Geometry: final body of the model. Coordinates: model frame, mm. Face numbers are marked on the shaded views. A direction names the side the tool comes from. Give positions to 0.01 mm unless a question says otherwise; leave off trailing zeros. Order: outer loops, then holes, each group sorted by start corner. A loop starts at its lowest first (then second) coordinate and runs counter-clockwise, first axis right, second up. Notation, with made-up numbers: M 79.25,-20 L 104.25,-20 A24 cw 104.25,12 Z; hole C -33,-0.5 d9. An arc over 180 degrees is marked long. Use CSV: the item, a comma, the result in double quotes.
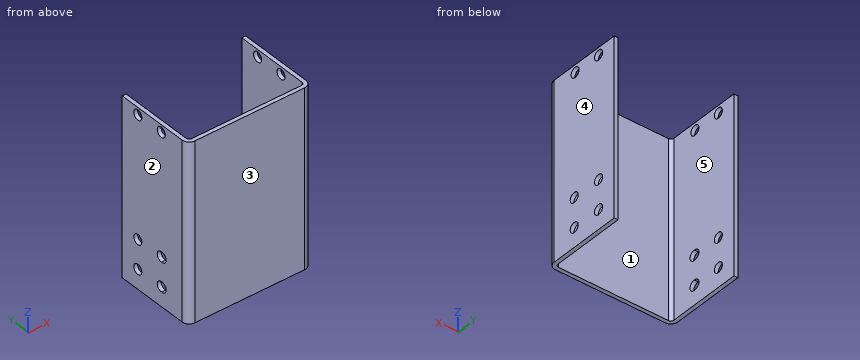
```python
from build123d import *

# Parameters (mm, degrees)
EXTRUDE_THIN1_DEPTH        = 57.935499968
F_4_CLEARANCE_HOLE1_REACH  = 115.405
F_4_CLEARANCE_HOLE1_BORE_R = 1.63195
F_4_CLEARANCE_HOLE2_D      = 3.2639
F_4_CLEARANCE_HOLE3_REACH  = 115.405
F_4_CLEARANCE_HOLE3_BORE_R = 1.63195
F_4_CLEARANCE_HOLE4_D      = 3.2639


with BuildPart() as part:
    # Sketch1 → Extrude-Thin1 (new body)
    with BuildSketch(Plane.XY):
        with BuildLine():
            Line((0, 25.4), (0, 1.016))
            ThreePointArc((0, 1.016), (0.29757951, 0.29757951), (1.016, 0))
            Line((1.016, 0), (37.084, 0))
            ThreePointArc((37.084, 0), (37.80242049, 0.29757951), (38.1, 1.016))
            Line((38.1, 1.016), (38.1, 25.4))
            Line((38.1, 25.4), (39.37, 25.4))
            Line((39.37, 25.4), (39.37, 1.016))
            ThreePointArc((39.37, 1.016), (38.700446102, -0.600446102), (37.084, -1.27))
            Line((37.084, -1.27), (1.016, -1.27))
            ThreePointArc((1.016, -1.27), (-0.600446102, -0.600446102), (-1.27, 1.016))
            Line((-1.27, 1.016), (-1.27, 25.4))
            Line((-1.27, 25.4), (0, 25.4))
        make_face()
    extrude(amount=EXTRUDE_THIN1_DEPTH)

    # #4 Clearance Hole1 bore → #4 Clearance Hole1 (cut, up to next)
    with BuildSketch(Plane(origin=(-1.27, -12.402043901, 98.894849861), x_dir=(0, 0, 1), z_dir=(-1, 0, 0)), mode=Mode.PRIVATE) as f_4_clearance_hole1_sk1:
        with Locations((-92.544849861, 31.452043901)):
            Circle(F_4_CLEARANCE_HOLE1_BORE_R)
    f_4_clearance_hole1_tool1 = extrude(f_4_clearance_hole1_sk1.sketch, amount=-F_4_CLEARANCE_HOLE1_REACH, mode=Mode.PRIVATE) & part.part
    # #4 Clearance Hole1 bore → #4 Clearance Hole1 (cut, up to next)
    with BuildSketch(Plane(origin=(-1.27, -12.402043901, 98.894849861), x_dir=(0, 0, 1), z_dir=(-1, 0, 0)), mode=Mode.PRIVATE) as f_4_clearance_hole1_sk2:
        with Locations((-83.019849861, 31.452043901)):
            Circle(F_4_CLEARANCE_HOLE1_BORE_R)
    f_4_clearance_hole1_tool2 = extrude(f_4_clearance_hole1_sk2.sketch, amount=-F_4_CLEARANCE_HOLE1_REACH, mode=Mode.PRIVATE) & part.part
    # #4 Clearance Hole1 bore → #4 Clearance Hole1 (cut, up to next)
    with BuildSketch(Plane(origin=(-1.27, -12.402043901, 98.894849861), x_dir=(0, 0, 1), z_dir=(-1, 0, 0)), mode=Mode.PRIVATE) as f_4_clearance_hole1_sk3:
        with Locations((-83.019849861, 21.927043901)):
            Circle(F_4_CLEARANCE_HOLE1_BORE_R)
    f_4_clearance_hole1_tool3 = extrude(f_4_clearance_hole1_sk3.sketch, amount=-F_4_CLEARANCE_HOLE1_REACH, mode=Mode.PRIVATE) & part.part
    # #4 Clearance Hole1 bore → #4 Clearance Hole1 (cut, up to next)
    with BuildSketch(Plane(origin=(-1.27, -12.402043901, 98.894849861), x_dir=(0, 0, 1), z_dir=(-1, 0, 0)), mode=Mode.PRIVATE) as f_4_clearance_hole1_sk4:
        with Locations((-92.544849861, 21.927043901)):
            Circle(F_4_CLEARANCE_HOLE1_BORE_R)
    f_4_clearance_hole1_tool4 = extrude(f_4_clearance_hole1_sk4.sketch, amount=-F_4_CLEARANCE_HOLE1_REACH, mode=Mode.PRIVATE) & part.part
    add(f_4_clearance_hole1_tool1.solids().sort_by_distance((-1.27, 19.05, 6.35))[0], mode=Mode.SUBTRACT)
    add(f_4_clearance_hole1_tool2.solids().sort_by_distance((-1.27, 19.05, 15.875))[0], mode=Mode.SUBTRACT)
    add(f_4_clearance_hole1_tool3.solids().sort_by_distance((-1.27, 9.525, 15.875))[0], mode=Mode.SUBTRACT)
    add(f_4_clearance_hole1_tool4.solids().sort_by_distance((-1.27, 9.525, 6.35))[0], mode=Mode.SUBTRACT)

    # #4 Clearance Hole2 (through all)
    with Locations(Plane(origin=(39.37, -12.402043901, 98.894849861), x_dir=(0, 0, -1), z_dir=(1, 0, 0))):
        with Locations((92.544849861, 31.452043901), (83.019849861, 31.452043901), (83.019849861, 21.57276521), (92.544849861, 21.57276521)):
            Hole(F_4_CLEARANCE_HOLE2_D / 2)

    # #4 Clearance Hole3 bore → #4 Clearance Hole3 (cut, up to next)
    with BuildSketch(Plane(origin=(-1.27, -12.402043901, 98.894849861), x_dir=(0, 0, 1), z_dir=(-1, 0, 0)), mode=Mode.PRIVATE) as f_4_clearance_hole3_sk1:
        with Locations((-43.372349893, 31.452043901)):
            Circle(F_4_CLEARANCE_HOLE3_BORE_R)
    f_4_clearance_hole3_tool1 = extrude(f_4_clearance_hole3_sk1.sketch, amount=-F_4_CLEARANCE_HOLE3_REACH, mode=Mode.PRIVATE) & part.part
    # #4 Clearance Hole3 bore → #4 Clearance Hole3 (cut, up to next)
    with BuildSketch(Plane(origin=(-1.27, -12.402043901, 98.894849861), x_dir=(0, 0, 1), z_dir=(-1, 0, 0)), mode=Mode.PRIVATE) as f_4_clearance_hole3_sk2:
        with Locations((-43.372349893, 21.927043901)):
            Circle(F_4_CLEARANCE_HOLE3_BORE_R)
    f_4_clearance_hole3_tool2 = extrude(f_4_clearance_hole3_sk2.sketch, amount=-F_4_CLEARANCE_HOLE3_REACH, mode=Mode.PRIVATE) & part.part
    add(f_4_clearance_hole3_tool1.solids().sort_by_distance((-1.27, 19.05, 55.5225))[0], mode=Mode.SUBTRACT)
    add(f_4_clearance_hole3_tool2.solids().sort_by_distance((-1.27, 9.525, 55.5225))[0], mode=Mode.SUBTRACT)

    # #4 Clearance Hole4 (through all)
    with Locations(Plane(origin=(39.37, -12.402043901, 98.894849861), x_dir=(0, 0, -1), z_dir=(1, 0, 0))):
        with Locations((43.372349893, 21.927043901), (43.372349893, 31.452043901)):
            Hole(F_4_CLEARANCE_HOLE4_D / 2)


solid = part.part
```
1. Reachability of the marked faces 4 and 5 from +Z, -Z, +X, -X, +Y, -Y: full face, straight path, thin tool, end or side. Return the list, or none.
Answer:
face 4,"+Z, -Z, +X, +Y, -Y"
face 5,"+Z, -Z, +Y"
2. Line query: line 1 (X direction, y = 13.5, z = 38); line 2 (Y direction, x = -0.3, z = 6.35); line 3 (Y direction, x = -1, z = 6.35). Output: solid intervals per line, ascending.
Answer:
line 1,"-1.27 to 0, 38.1 to 39.37"
line 2,"-0.85 to 7.54, 11.16 to 17.42, 20.68 to 25.4"
line 3,"-0.06 to 7.54, 11.16 to 17.42, 20.68 to 25.4"
3. Section B-B, the plane z = 6.35. Return the cut outline in (x, y), plus the area to 3 significant figures.
Answer:
outline,"M -1.27,1.02 A2.29 ccw 1.02,-1.27 L 37.08,-1.27 A2.29 ccw 39.37,1.02 L 39.37,7.54 L 38.1,7.54 L 38.1,1.02 A1.02 cw 37.08,0 L 1.02,0 A1.02 cw 0,1.02 L 0,7.54 L -1.27,7.54 Z; M -1.27,11.16 L 0,11.16 L 0,17.42 L -1.27,17.42 Z; M -1.27,20.68 L 0,20.68 L 0,25.4 L -1.27,25.4 Z; M 38.1,10.8 L 39.37,10.8 L 39.37,17.42 L 38.1,17.42 Z; M 38.1,20.68 L 39.37,20.68 L 39.37,25.4 L 38.1,25.4 Z"
area,"97.3 mm2"
4. Section D-D, the plane z = 46. Return the cut outline in (x, y).
Answer:
outline,"M -1.27,1.02 A2.29 ccw 1.02,-1.27 L 37.08,-1.27 A2.29 ccw 39.37,1.02 L 39.37,25.4 L 38.1,25.4 L 38.1,1.02 A1.02 cw 37.08,0 L 1.02,0 A1.02 cw 0,1.02 L 0,25.4 L -1.27,25.4 Z"
5. Section C-C, the plane y = 19.05. Give the number of separate pieces and of enclosed holes in the cut face, plus the area to 3 significant figures.
Answer:
separate pieces,"8"
enclosed holes,"0"
area,"122 mm2"
6. Pull-direction query (X, two-part tool) for the marked faces 1, 2 and 3; classes: +X half, -X half, draft (parallel to the pull), parting line (faces both ways), or undercut.
Answer:
face 1,"undercut"
face 2,"-X half"
face 3,"draft"
7. Section A-A, the plane y = 13.75. Return the cut outline in (x, z), plus the area to 3 significant figures.
Answer:
outline,"M -1.27,0 L 0,0 L 0,57.94 L -1.27,57.94 Z; M 38.1,0 L 39.37,0 L 39.37,57.94 L 38.1,57.94 Z"
area,"147 mm2"
